from build123d import *

# Parameters (mm, degrees)
SKETCH1_W                 = 33
SKETCH1_H                 = 33
SKETCH1_R                 = 2
BOSS_EXTRUDE1_DEPTH       = 1.6
SKETCH2_W                 = 16
SKETCH2_H                 = 16
BOSS_EXTRUDE2_DEPTH       = 10
BOSS_EXTRUDE3_START       = -10
BOSS_EXTRUDE3_DEPTH       = 10
SKETCH4_R                 = 7.5
SKETCH4_R_2               = 5.5
BOSS_EXTRUDE4_DEPTH       = 3
CUT_EXTRUDE1_START        = -8
SKETCH5_R                 = 5.5
CUT_EXTRUDE1_DEPTH        = 8
SKETCH7_R                 = 0.2
LPATTERN1_COUNT           = 2
LPATTERN1_PITCH           = 3
SKETCH8_R                 = 2.75
BOSS_EXTRUDE7_DEPTH       = 0.7
SKETCH9_R                 = 2.5
BOSS_EXTRUDE8_DEPTH       = 7
FILLET1_R                 = 2.5
LPATTERN2_COUNT           = 2
LPATTERN2_PITCH           = 12
LPATTERN2_COPY_1_SKETCH_R = 0.2
FILLET1_OF_LPATTERN2_R    = 2.5


# Read off the part's stored shape, not the designer's step: Mirror1
with BuildPart() as part:
    # Sketch1 → Boss-Extrude1 (new body)
    with BuildSketch(Plane(origin=(0, 0, 0), x_dir=(1, 0, 0), z_dir=(0, 1, 0))):
        Rectangle(SKETCH1_W, SKETCH1_H)
        with Locations(Location((-12.5, 12.5, 0), (0, 0, 270))):
            Circle(SKETCH1_R, mode=Mode.SUBTRACT)
        with Locations(Location((12.5, 12.5, 0), (0, 0, 270))):
            Circle(SKETCH1_R, mode=Mode.SUBTRACT)
        with Locations(Location((12.5, -12.5, 0), (0, 0, 270))):
            Circle(SKETCH1_R, mode=Mode.SUBTRACT)
        with Locations(Location((-12.5, -12.5, 0), (0, 0, 270))):
            Circle(SKETCH1_R, mode=Mode.SUBTRACT)
    extrude(amount=BOSS_EXTRUDE1_DEPTH)

    # Sketch2 → Boss-Extrude2 (add)
    with BuildSketch(Plane(origin=(0, 1.6, 0), x_dir=(1, 0, 0), z_dir=(0, 1, 0))):
        Rectangle(SKETCH2_W, SKETCH2_H)
    extrude(amount=BOSS_EXTRUDE2_DEPTH)

    # Sketch3 → Boss-Extrude3 (add)
    with BuildSketch(Plane(origin=(0, 11.6, 0), x_dir=(1, 0, 0), z_dir=(0, 1, 0)).offset(BOSS_EXTRUDE3_START)):
        with BuildLine():
            Line((-1.5, -10), (-1.5, 10))
            ThreePointArc((-1.5, 10), (0, 11.5), (1.5, 10))
            Line((1.5, 10), (1.5, -10))
            ThreePointArc((1.5, -10), (0, -11.5), (-1.5, -10))
        make_face()
    extrude(amount=BOSS_EXTRUDE3_DEPTH)

    # Sketch4 → Boss-Extrude4 (add)
    with BuildSketch(Plane(origin=(0, 11.6, 0), x_dir=(1, 0, 0), z_dir=(0, 1, 0))):
        with Locations(Location((0, 0, 0), (0, 0, 90))):
            Circle(SKETCH4_R)
        with Locations(Location((0, 0, 0), (0, 0, 270))):
            Circle(SKETCH4_R_2, mode=Mode.SUBTRACT)
    extrude(amount=BOSS_EXTRUDE4_DEPTH)

    # Sketch5 → Cut-Extrude1 (cut)
    with BuildSketch(Plane(origin=(0, 11.6, 0), x_dir=(1, 0, 0), z_dir=(0, 1, 0)).offset(CUT_EXTRUDE1_START)):
        with Locations(Location((0, 0, 0), (0, 0, 270))):
            Circle(SKETCH5_R)
    extrude(amount=CUT_EXTRUDE1_DEPTH, mode=Mode.SUBTRACT)

    # Sweep1: sweep along a path in Sketch6
    with BuildLine(Plane.ZY.offset(7.5)) as sweep1_path:
        Line((-11.5, 1.6), (-7.357383869, 21.166265142))
    # Sketch7 → Sweep1 (sweep)
    with BuildSketch(Plane(origin=(-7.5, 21.166265142, -7.357383869), x_dir=(1, 0, 0), z_dir=(0, 0.9783132570757084, 0.2071308065689869))):
        Circle(SKETCH7_R)
    sweep1 = sweep(path=sweep1_path.line)

    # LPattern1: Sweep1 ×2
    with Locations(*[(i * LPATTERN1_PITCH, 0, 0) for i in range(1, LPATTERN1_COUNT)]):
        add(sweep1)

    # Sketch8 → Boss-Extrude7 (add)
    with BuildSketch(Plane(origin=(0, 18.767273707, 3.973451767), x_dir=(1, 0, 0), z_dir=(0, 0.9783132570757084, 0.20713080656898694))):
        with Locations(Location((-6, 11.582011747, 0), (0, 0, 270))):
            Circle(SKETCH8_R)
    boss_extrude7 = extrude(amount=-BOSS_EXTRUDE7_DEPTH)

    # Sketch9 → Boss-Extrude8 (add)
    with BuildSketch(Plane(origin=(0, 18.767273707, 3.973451767), x_dir=(1, 0, 0), z_dir=(0, 0.9783132570757084, 0.20713080656898694))):
        with Locations(Location((-6, 11.582011747, 0), (0, 0, 270))):
            Circle(SKETCH9_R)
    boss_extrude8 = extrude(amount=BOSS_EXTRUDE8_DEPTH)

    # Fillet1
    fillet1_edges = [part.edges().sort_by_distance(p)[0] for p in [
        (-6, 28.532284957, -8.353251365),
    ]]
    fillet(fillet1_edges, radius=FILLET1_R)

    # LPattern2: Sweep1, Boss-Extrude7, Boss-Extrude8 ×2
    with Locations(*[(i * LPATTERN2_PITCH, 0, 0) for i in range(1, LPATTERN2_COUNT)]):
        add(sweep1)
        add(boss_extrude7)
        add(boss_extrude8)

    # LPattern2 copy 1: sweep along a path in LPattern2 copy 1 path
    with BuildLine(Plane.ZY.offset(-7.5)) as lpattern2_copy_1_path:
        Line((-11.5, 1.6), (-7.357383869, 21.166265142))
    # LPattern2 copy 1 sketch → LPattern2 copy 1 (sweep)
    with BuildSketch(Plane(origin=(7.5, 21.166265142, -7.357383869), x_dir=(1, 0, 0), z_dir=(0, 0.9783132570757084, 0.2071308065689869))):
        Circle(LPATTERN2_COPY_1_SKETCH_R)
    sweep(path=lpattern2_copy_1_path.line)

    # Fillet1 of LPattern2
    fillet1_of_lpattern2_edges = [part.edges().sort_by_distance(p)[0] for p in [
        (6, 28.532284957, -8.353251365),
    ]]
    fillet(fillet1_of_lpattern2_edges, radius=FILLET1_OF_LPATTERN2_R)

    # Mirror1: part across plane


with BuildPart() as part_1:
    add(part.part)
    add(part.part.mirror(Plane.XY))


solid = part_1.part
Work out the finished part from the listing and answer in its coordinate system (mm). A direction names the side the tool comes from. Give positions to 0.01 mm unless a question says otherwise; leave off trailing zeros. Loops run counter-clockwise (first coordinate to the right, second up) from the corner with the lowest first, then second, coordinate; pieces in that order, holes last. Notation, with made-up numbers: (-17.5, 35.5) - (-10.5, 35.5) arc R15 ccw to (-10.5, 57.5) - close; hole circle Ø3 at (83, 33.25). An arc over 180 degrees is marked (long way). Answer in a Markdown table with one row per item. Add a question column.
Q1. Determine the mould class of faces 1 (the cylindrical face through (7.69, 11.19, 9.53)), 2 (the flat face through (0, 3.6, 0)), 3 (the cylindrical face through (0, 6.5, 11.5)) for opening direction Y: released by +Y, released by -Y, zero draft, split by the parting line, or undercut.
Q2. The part is cut by section B-B (x = 6.5). Determine the outline of the cut face in (y, z), and give its area (3 significant figures).
Q3. The part is cut by section C-C (z = 0). Determine the outline of the cut face in (x, y).
Q4. Each of these flat-tipped pins is pushed along its axis until it touches: P1, Ø5, axis at y = 5, z = 0.5, coming from the +X side; P2, Ø4.5, axis at x = -12.5, z = 12.5, coming from the +Y side; P3, Ø7, axis at x = -3.5, y = 5.5, coming from the -Z side; P4, Ø3, axis at x = -12.5, z = -12.5, coming from the +Y side. Where does it stop, or does it pass through?
Q5. The part is cut by section A-A (z = 12.5). Determine the outline of the cut face in (x, y), and give its area (3 significant figures).
Q6. The part is cut by section D-D (x = 0). Determine the outline of the cut face in (y, z), and give its area (3 significant figures).
Q7. A tool of negligible diameter and unlimited length cuts with its end or side. For faces 4 (the flat face through (0, 1, 16.5)), 5 (the flat face through (1, 11.6, 8)), from which of +Z, -Z, +X, -X, +Y, -Y can it reach the whole face along a straight path? Write none if from no direction.
Q8. Consider line 1 along X through (y, z) = (0.95, 12.5); line 2 along X through (y, z) = (8.5, 0). Determine where each line is inside the solid, lowest interval first.
Solution:
| question | item | result |
|---|---|---|
| 1 | face 1 | undercut |
| 1 | face 2 | released by +Y |
| 1 | face 3 | zero draft |
| 2 | outline | (0, -16.5) - (1.6, -16.5) - (1.6, -8) - (11.6, -8) - (11.6, -3.74) - (14.6, -3.74) - (14.6, 3.74) - (11.6, 3.74) - (11.6, 8) - (1.6, 8) - (1.6, 16.5) - (0, 16.5) - close; (19.92, -4.86) - (21.04, -10.15) - (21.73, -10) - (21.67, -9.75) - (26.08, -8.82) arc R2.45 ccw to (25.06, -4.03) - (20.66, -4.96) - (20.61, -4.71) - close; (19.92, 4.86) - (20.61, 4.71) - (20.66, 4.96) - (25.06, 4.03) arc R2.45 ccw to (26.08, 8.82) - (21.67, 9.75) - (21.73, 10) - (21.04, 10.15) - close |
| 2 | area | 306 mm² |
| 3 | outline | (-16.5, 0) - (16.5, 0) - (16.5, 1.6) - (8, 1.6) - (8, 11.6) - (7.5, 11.6) - (7.5, 14.6) - (5.5, 14.6) - (5.5, 3.6) - (-5.5, 3.6) - (-5.5, 14.6) - (-7.5, 14.6) - (-7.5, 11.6) - (-8, 11.6) - (-8, 1.6) - (-16.5, 1.6) - close |
| 4 | P1 | stops at x = 8 |
| 4 | P2 | stops at y = 1.6 |
| 4 | P3 | stops at z = -11.59 |
| 4 | P4 | passes through |
| 5 | outline | (-16.5, 0) - (-14.5, 0) - (-14.5, 1.6) - (-16.5, 1.6) - close; (-10.5, 0) - (10.5, 0) - (10.5, 1.6) - (-10.5, 1.6) - close; (14.5, 0) - (16.5, 0) - (16.5, 1.6) - (14.5, 1.6) - close |
| 5 | area | 40.0 mm² |
| 6 | outline | (0, -16.5) - (1.6, -16.5) - (1.6, -11.5) - (11.6, -11.5) - (11.6, -7.5) - (14.6, -7.5) - (14.6, -5.5) - (3.6, -5.5) - (3.6, 5.5) - (14.6, 5.5) - (14.6, 7.5) - (11.6, 7.5) - (11.6, 11.5) - (1.6, 11.5) - (1.6, 16.5) - (0, 16.5) - close |
| 6 | area | 207 mm² |
| 7 | face 4 | +Z, +X, -X, +Y, -Y |
| 7 | face 5 | none |
| 8 | line 1 | x = -16.5 to -14.5, -10.5 to 10.5, 14.5 to 16.5 |
| 8 | line 2 | x = -8 to -5.5, 5.5 to 8 |
